Design review of the part built by this model. Coordinates are the model's own, in mm. A direction names the side the tool comes from. Round coordinates to 2 decimals unless told otherwise and drop trailing zeros. Write item = value, one per line.
from build123d import *

# Parameters (mm, degrees)
F0_W     = 20
F0_H     = 40
F1_DEPTH = 850
F2_R     = 2.5
F3_DEPTH = 20
F4_W     = 10
F4_H     = 20
F4_W_2   = 10.3488773853
F5_DEPTH = 500


with BuildPart() as f1:
    # F0 (on Top) → F1 (new body)
    with BuildSketch(Plane.XY):
        Rectangle(F0_W, F0_H)
    extrude(amount=F1_DEPTH)

    # F2 (on face) → F3 (cut)
    with BuildSketch(Plane(origin=(0, 20, 0), x_dir=(-1, 0, 0), z_dir=(0, 1, 0))):
        with Locations((0, 555)):
            Circle(F2_R)
        with Locations((0, 705)):
            Circle(F2_R)
        with Locations((0, 255)):
            Circle(F2_R)
        with Locations((0, 105)):
            Circle(F2_R)
        with Locations((0, 405)):
            Circle(F2_R)
    extrude(amount=-F3_DEPTH, mode=Mode.SUBTRACT)

    # F4 (on face) → F5 (cut)
    with BuildSketch(Plane.YZ.offset(10)):
        with Locations((-15, 840)):
            Rectangle(F4_W, F4_H)
        with Locations((15, 840)):
            Rectangle(F4_W, F4_H)
        with Locations((14.8255613074, 10)):
            Rectangle(F4_W_2, F4_H)
        with Locations((-15, 10)):
            Rectangle(F4_W, F4_H)
    extrude(amount=-F5_DEPTH, mode=Mode.SUBTRACT)


solid = f1.part
1) To check wall thickness, follow L1, parallel to Z at x = 0, y = 9.75; L2, parallel to Z at x = 0, y = 7.5; L3, parallel to X at y = 5.5, z = 405. State the ranges of each line that lie inside material, in increasing order. Write a range as from..to.
Findings:
L1 = 20..102.5, 107.5..252.5, 257.5..402.5, 407.5..552.5, 557.5..702.5, 707.5..850
L2 = 0..102.5, 107.5..252.5, 257.5..402.5, 407.5..552.5, 557.5..702.5, 707.5..850
L3 = -10..-2.5, 2.5..10
2) Clearance check with flat-ended pins moving along their axes: pin 1 Ø3 at (x, y) = (-3, -13.5) entering from -Z; pin 2 Ø10 at (x, z) = (3, 836.5) entering from +Y; pin 3 Ø3 at (x, z) = (0, 705) entering from +Y. State where each tip first meets the part, or that it passes through.
Findings:
pin_1 = 20
pin_2 = 10
pin_3 = 0
3) For faces 1 (the flat face through (0, 9.651, 10)), 2 (the flat face through (0, -10, 10)), 3 (the flat face through (0, 10, 840)), 4 (the flat face through (0, -10, 840)), list the 3-axis set-ups (+Z, -Z, +X, -X, +Y, -Y) from which the entire face can be reached by the end or side of a thin tool; tool diameter is ignored.
Findings:
face_1 = -Z, +X, -X, +Y
face_2 = -Z, +X, -X, -Y
face_3 = +Z, +X, -X, +Y
face_4 = +Z, +X, -X, -Y
